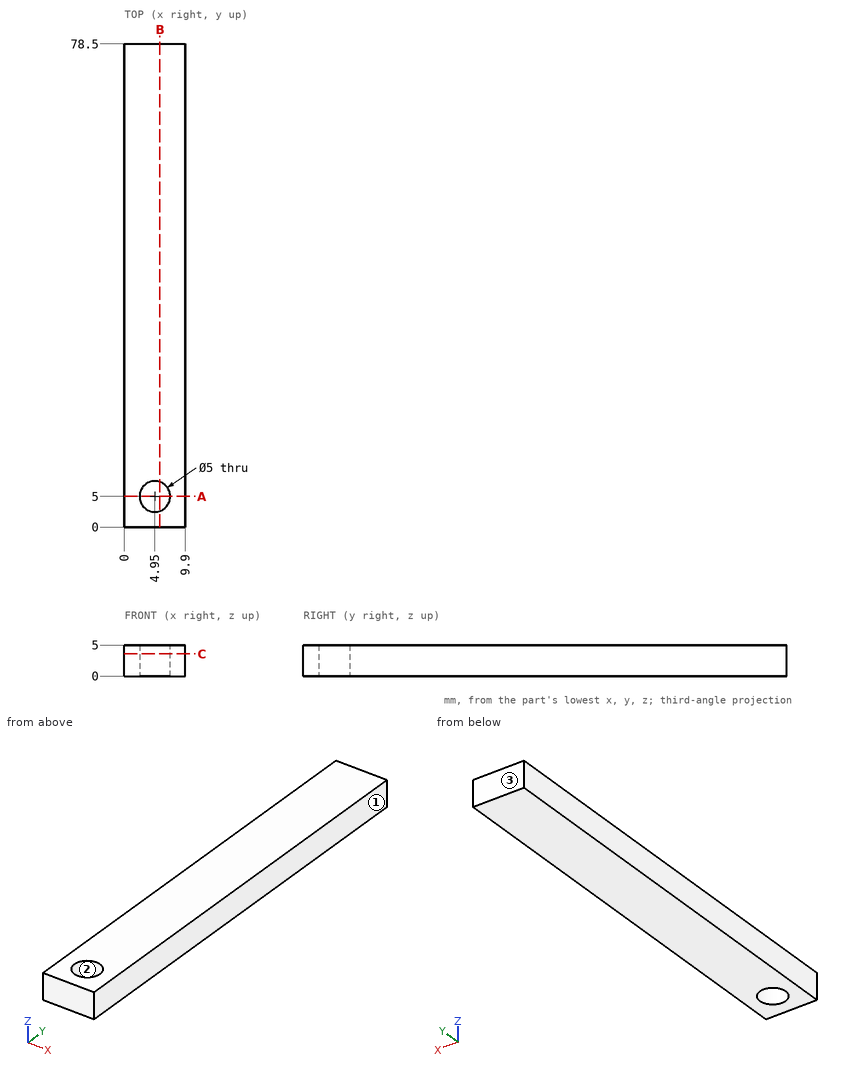
Answer from the drawing. Dimensions are ordinates in mm from the lowest x, y and z of the part. Round coordinates to 2 decimals unless told otherwise and drop trailing zeros. Loops run counter-clockwise (first coordinate to the right, second up) from the corner with the lowest first, then second, coordinate; pieces in that order, holes last.
(1) The part is cut by section A-A, the plane y = 5. Give the vertices of the cut face in (x, z).
Computed values:
outline: (0, 0) - (2.45, 0) - (2.45, 5) - (0, 5) - close; (7.45, 0) - (9.9, 0) - (9.9, 5) - (7.45, 5) - close
(2) Find the intervals of material crossed by L1, parallel to Y at x = 4.95, z = 3.1; L2, parallel to X at y = 7, z = 1.05, in increasing order.
Computed values:
L1: y = 0 to 2.5, 7.5 to 78.5
L2: x = 0 to 3.45, 6.45 to 9.9
(3) The part is cut by section C-C, the plane z = 3.6. Give the vertices of the cut face in (x, y), and give its area (3 significant figures).
Computed values:
outline: (0, 0) - (9.9, 0) - (9.9, 78.5) - (0, 78.5) - close; hole circle Ø5 at (4.95, 5)
area: 758 mm2
(4) The mould has two halves that part along Y. Classify the marked faces 1, 2 and 3: pulls with the +Y half, pulls with the -Y half, needs draft (parallel to the pull), parting line crosses it, or undercut.
Computed values:
face 1: needs draft
face 2: undercut
face 3: pulls with the +Y half
(5) The part is cut by section B-B, the plane x = 5.75. Give the vertices of the cut face in (y, z), and give its area (3 significant figures).
Computed values:
outline: (0, 0) - (2.63, 0) - (2.63, 5) - (0, 5) - close; (7.37, 0) - (78.5, 0) - (78.5, 5) - (7.37, 5) - close
area: 369 mm2
